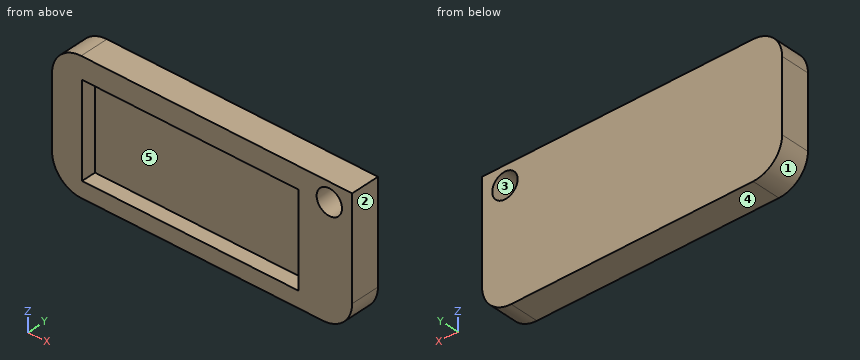
```python
from build123d import *

# Parameters (mm, degrees)
F0_W     = 47.305181
F0_H     = 20.148503
F1_DEPTH = 6.35
F2_DEPTH = 3.175
F3_R     = 2.767863
F4_DEPTH = 25.4


with BuildPart() as f1:
    # F0 (on Front) → F1 (new body)
    with BuildSketch(Plane.XZ):
        with BuildLine():
            Line((65.55564, 35.770893), (6.35, 35.770893))
            ThreePointArc((6.35, 35.770893), (1.859872, 33.911021), (0, 29.420893))
            Line((0, 29.420893), (0, 13.796186))
            ThreePointArc((0, 13.796186), (1.859872, 9.306058), (6.35, 7.446186))
            Line((6.35, 7.446186), (59.20564, 7.446186))
            ThreePointArc((59.20564, 7.446186), (63.695768, 9.306058), (65.55564, 13.796186))
            Line((65.55564, 13.796186), (65.55564, 35.770893))
        make_face()
        with Locations((30.222755, 21.024525)):
            Rectangle(F0_W, F0_H, mode=Mode.SUBTRACT)
    extrude(amount=F1_DEPTH)

    # F0 (on Front) → F2 (join)
    with BuildSketch(Plane.XZ):
        with Locations((30.222755, 21.024525)):
            Rectangle(F0_W, F0_H)
    extrude(amount=F2_DEPTH)

    # F3 (on face) → F4 (cut)
    with BuildSketch(Plane.XZ.offset(6.35)):
        with Locations((60.560498, 31.713862)):
            Circle(F3_R)
    extrude(amount=-F4_DEPTH, mode=Mode.SUBTRACT)


solid = f1.part
```
Input: part model. Units: mm. Frame: model coordinates. Face numbers are marked on the shaded views. A direction names the side the tool comes from. Give positions to 0.01 mm unless a question says otherwise; leave off trailing zeros. Order: outer loops, then holes, each group sorted by start corner. A loop starts at its lowest first (then second) coordinate and runs counter-clockwise, first axis right, second up.
1. Section D-D on y = -5. Return the cut outline in (x, z).
Derived:
outline: (0, 13.8) arc R6.35 ccw to (6.35, 7.45) - (59.21, 7.45) arc R6.35 ccw to (65.56, 13.8) - (65.56, 35.77) - (6.35, 35.77) arc R6.35 ccw to (0, 29.42) - close; hole (6.57, 10.95) - (53.88, 10.95) - (53.88, 31.1) - (6.57, 31.1) - close; hole circle Ø5.54 at (60.56, 31.71)
2. Section A-A on y = -2.25. Return the cut outline in (x, z), and give its area (3 significant figures).
Derived:
outline: (0, 13.8) arc R6.35 ccw to (6.35, 7.45) - (59.21, 7.45) arc R6.35 ccw to (65.56, 13.8) - (65.56, 35.77) - (6.35, 35.77) arc R6.35 ccw to (0, 29.42) - close; hole circle Ø5.54 at (60.56, 31.71)
area: 1,810 mm2
3. Section B-B on x = 43. Return the cut outline in (y, z) (3 decimals), and give its area (3 significant figures).
Derived:
outline: (-6.35, 7.446) - (0, 7.446) - (0, 35.771) - (-6.35, 35.771) - (-6.35, 31.099) - (-3.175, 31.099) - (-3.175, 10.95) - (-6.35, 10.95) - close
area: 116 mm2
4. Section C-C on z = 32.75. Return the cut outline in (x, y).
Derived:
outline: (0.94, -6.35) - (57.99, -6.35) - (57.99, 0) - (0.94, 0) - close; (63.13, -6.35) - (65.56, -6.35) - (65.56, 0) - (63.13, 0) - close
5. Mould query, pull axis Z, two halves, no side actions, for the marked faces 1, 2 and 3. Classes: released by +Z, released by -Z, zero draft, split by the parting line, or undercut.
Derived:
face 1: released by -Z
face 2: zero draft
face 3: undercut
6. Material intervals for L1, parallel to Z at x = 21.5, y = -4.25; L2, parallel to X at y = -3.75, z = 23.25; L3, parallel to Y at x = 52, z = 26.5 (3 decimals), sorted ascending.
Derived:
L1: z = 7.45 to 10.95, 31.1 to 35.77
L2: x = 0 to 6.57, 53.88 to 65.56
L3: y = -3.175 to 0
7. Reachability of the marked faces 4 and 5 from +Z, -Z, +X, -X, +Y, -Y: full face, straight path, thin tool, end or side. Return the list, or none.
Derived:
face 4: -Z, +X, -X, +Y, -Y
face 5: -Y
8. Pin query (flat end, axial travel): pin 1 (4.5 mm diameter, centred on x = 60.56, z = 31.71, fed in from +Y); pin 2 (10 mm diameter, centred on x = 46, z = 11.5, fed in from -Y); pin 3 (6 mm diameter, centred on x = 21, z = 21, fed in from -Y) (3 decimals). Return the tip coordinate at first contact, or that it passes through.
Derived:
pin 1: passes through
pin 2: stops at y = -6.35
pin 3: stops at y = -3.175
